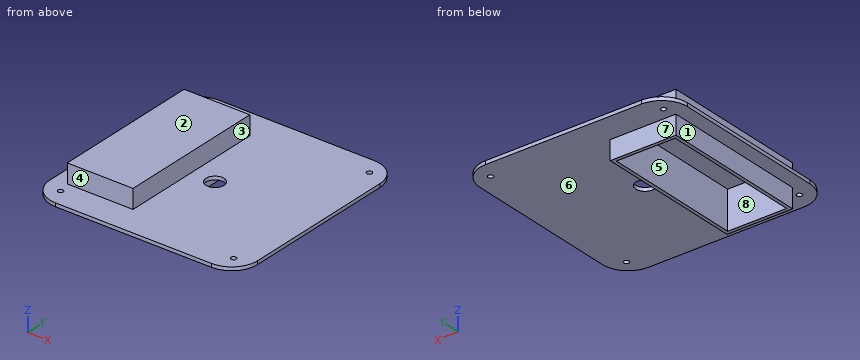
from build123d import *

# Parameters (mm, degrees)
F2_W     = 38
F2_H     = 86
F2_W_2   = 34
F2_H_2   = 82
F3_DEPTH = 13
F4_DEPTH = 11
F5_DEPTH = 11
F2_R     = 1.5
F2_R_2   = 5.25
F6_DEPTH = 2


with BuildPart() as f3:
    # F2 (on Top) → F3 (new body)
    with BuildSketch(Plane.XY):
        with Locations((-82.4976554215, 68.799585104)):
            Rectangle(F2_W, F2_H)
        with Locations((-82.4976554215, 68.799585104)):
            Rectangle(F2_W_2, F2_H_2, mode=Mode.SUBTRACT)
        with Locations((-82.4976554215, 68.799585104)):
            Rectangle(F2_W_2, F2_H_2)
    extrude(amount=F3_DEPTH)

    # F2 (on Top) → F4 (cut)
    with BuildSketch(Plane.XY):
        with Locations((-82.4976554215, 68.799585104)):
            Rectangle(F2_W_2, F2_H_2)
    extrude(amount=F4_DEPTH, mode=Mode.SUBTRACT)

    # F2 (on Top) → F5 (join)
    with BuildSketch(Plane.XY):
        with Locations((-82.4976554215, 68.799585104)):
            Rectangle(F2_W, F2_H)
        with Locations((-82.4976554215, 68.799585104)):
            Rectangle(F2_W_2, F2_H_2, mode=Mode.SUBTRACT)
    extrude(amount=-F5_DEPTH)

    # F2 (on Top) → F6 (join)
    with BuildSketch(Plane.XY):
        with BuildLine():
            Line((-94.8726554215, 8.799585104), (-4.8726554215, 8.799585104))
            ThreePointArc((-4.8726554215, 8.799585104), (5.7339462963, 13.1929833862), (10.1273445785, 23.799585104))
            Line((10.1273445785, 23.799585104), (10.1273445785, 113.799585104))
            ThreePointArc((10.1273445785, 113.799585104), (5.7339462963, 124.4061868218), (-4.8726554215, 128.799585104))
            Line((-4.8726554215, 128.799585104), (-94.8726554215, 128.799585104))
            ThreePointArc((-94.8726554215, 128.799585104), (-105.4792571393, 124.4061868218), (-109.8726554215, 113.799585104))
            Line((-109.8726554215, 113.799585104), (-109.8726554215, 23.799585104))
            ThreePointArc((-109.8726554215, 23.799585104), (-105.4792571393, 13.1929833862), (-94.8726554215, 8.799585104))
        make_face()
        with Locations((-99.8726554215, 18.799585104)):
            Circle(F2_R, mode=Mode.SUBTRACT)
        with Locations((0.1273445785, 18.799585104)):
            Circle(F2_R, mode=Mode.SUBTRACT)
        with Locations((-82.4976554215, 68.799585104)):
            Rectangle(F2_W, F2_H, mode=Mode.SUBTRACT)
        with Locations((-49.8726554215, 68.799585104)):
            Circle(F2_R_2, mode=Mode.SUBTRACT)
        with Locations((-99.8726554215, 118.799585104)):
            Circle(F2_R, mode=Mode.SUBTRACT)
        with Locations((0.1273445785, 118.799585104)):
            Circle(F2_R, mode=Mode.SUBTRACT)
    extrude(amount=F6_DEPTH)


solid = f3.part
Verification items for the finished model (mm, model axes). Face numbers are marked on the shaded views. A direction names the side the tool comes from. Give positions to 0.01 mm unless a question says otherwise; leave off trailing zeros. Write each loop counter-clockwise with the first axis right and the second up, starting at its lowest first coordinate (ties: lowest second). Pieces come first, ordered by that corner, then holes. Notation, with made-up numbers: M 0,-2 L 33,-2 A16 cw 33,8 Z; hole C -3.75,36 d10. An arc over 180 degrees is marked long. Write item = value, one per line.
(1) Access from +Z, -Z, +X, -X, +Y, -Y to the whole of each face (thin tool, end or side, straight path). Record for the marked faces 1, 2, 3, 4 and 5.
Found:
face_1 = -Z, -X, +Y, -Y
face_2 = +Z, +X, -X, +Y, -Y
face_3 = +Z, +X, +Y, -Y
face_4 = +Z, +X, -X, -Y
face_5 = -Z
(2) Material ranges on line 1 (X direction, y = 34, z = 4.75); line 2 (X direction, y = 28, z = 1); line 3 (Y direction, x = -84, z = 4.75), recorded low to high.
Found:
line_1 = -101.5 to -99.5, -65.5 to -63.5
line_2 = -109.87 to -99.5, -65.5 to 10.13
line_3 = 25.8 to 27.8, 109.8 to 111.8
(3) Go/stop test with flat-tipped pins: pin 1 Ø3.5 at (y, z) = (54.5, 6.5) entering from +X; pin 2 Ø8 at (x, y) = (-51, 96) entering from -Z; pin 3 Ø2 at (x, y) = (-20, 71) entering from +Z. Record where each tip stops, or that it passes through.
Found:
pin_1 = -63.5
pin_2 = 0
pin_3 = 2
(4) Sectioned sample at D-D (x = -84). Record the cut outline in (y, z), then the cut area to 3 significant figures.
Found:
outline = M 8.8,0 L 25.8,0 L 25.8,-11 L 27.8,-11 L 27.8,11 L 109.8,11 L 109.8,-11 L 111.8,-11 L 111.8,0 L 128.8,0 L 128.8,2 L 111.8,2 L 111.8,13 L 25.8,13 L 25.8,2 L 8.8,2 Z
area = 328 mm2
(5) Sectioned sample at B-B (z = 4). Record the cut outline in (x, y).
Found:
outline = M -101.5,25.8 L -63.5,25.8 L -63.5,111.8 L -101.5,111.8 Z; hole M -99.5,27.8 L -65.5,27.8 L -65.5,109.8 L -99.5,109.8 Z
(6) Sectioned sample at A-A (y = 57). Record the cut outline in (x, z).
Found:
outline = M -109.87,0 L -101.5,0 L -101.5,-11 L -99.5,-11 L -99.5,11 L -65.5,11 L -65.5,-11 L -63.5,-11 L -63.5,0 L 10.13,0 L 10.13,2 L -63.5,2 L -63.5,13 L -101.5,13 L -101.5,2 L -109.87,2 Z
(7) Sectioned sample at C-C (x = -48.5). Record the cut outline in (y, z), then the cut area to 3 significant figures.
Found:
outline = M 8.8,0 L 63.73,0 L 63.73,2 L 8.8,2 Z; M 73.87,0 L 128.8,0 L 128.8,2 L 73.87,2 Z
area = 220 mm2
(8) Draft check along Y on the marked faces 6, 7 and 8. Enter one of: released by +Y, released by -Y, zero draft, split by the parting line, or undercut.
Found:
face_6 = zero draft
face_7 = released by +Y
face_8 = undercut
